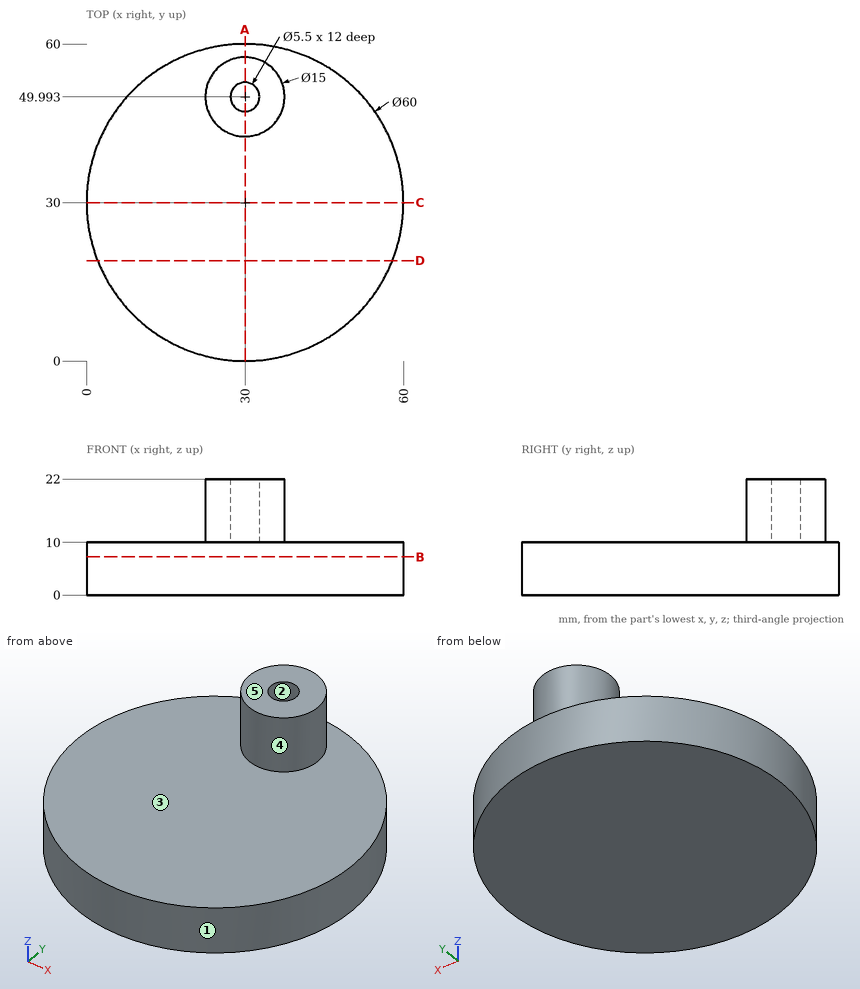
Answer from the drawing. Dimensions are ordinates in mm from the lowest x, y and z of the part. A direction names the side the tool comes from. Give positions to 0.01 mm unless a question says otherwise; leave off trailing zeros. Order: outer loops, then holes, each group sorted by start corner. A loop starts at its lowest first (then second) coordinate and runs counter-clockwise, first axis right, second up.
(1) Given pin 1 (5 mm diameter, centred on y = 32.5, z = 4, fed in from -X); pin 2 (4.5 mm diameter, centred on x = 30, y = 49.99, fed in from +Z); pin 3 (5 mm diameter, centred on y = 45.5, z = 7.5, fed in from -X); pin 4 (8 mm diameter, centred on y = 12, z = 4, fed in from -X), each flat-ended and moving along its own axis, determine where each tip first touches the part or whether it passes through.
(2) For a pull along Y with two mould halves and no side action, classify the marked faces 1, 2 and 3 as released by +Y, released by -Y, zero draft, split by the parting line, or undercut.
(3) Find section C-C (y = 30). Give the vertices of the cut face in (x, z).
(4) Find section D-D (y = 19). Give the vertices of the cut face in (x, z).
(5) Find section B-B (z = 7.25). Give the vertices of the cut face in (x, y), plus the area to 3 significant figures.
(6) Straight lines are drawn through the part: L1, parallel to Y at x = 30, z = 17; L2, parallel to Z at x = 34, y = 6.5; L3, parallel to X at y = 48, z = 18.75 (1 decimal). For each, find the intervals that lie inside material, in ascending order.
(7) Find section A-A (x = 30). Give the vertices of the cut face in (y, z).
(8) For the marked faces 4 and 5, determine the directions among +Z, -Z, +X, -X, +Y, -Y from which every point of the face is accessible in a straight line to the end or side of a thin tool.
Result sheet:
1. pin 1: stops at x = 0
1. pin 2: stops at z = 10
1. pin 3: stops at x = 2.96
1. pin 4: stops at x = 3.47
2. face 1: split by the parting line
2. face 2: undercut
2. face 3: zero draft
3. outline: (0, 0) - (60, 0) - (60, 10) - (0, 10) - close
4. outline: (2.09, 0) - (57.91, 0) - (57.91, 10) - (2.09, 10) - close
5. outline: circle Ø60 at (30, 30)
5. area: 2,830 mm2
6. L1: y = 42.49 to 47.24, 52.74 to 57.49
6. L2: z = 0 to 10
6. L3: x = 22.8 to 28.1, 31.9 to 37.2
7. outline: (0, 0) - (60, 0) - (60, 10) - (57.49, 10) - (57.49, 22) - (52.74, 22) - (52.74, 10) - (47.24, 10) - (47.24, 22) - (42.49, 22) - (42.49, 10) - (0, 10) - close
8. face 4: +Z
8. face 5: +Z, +X, -X, +Y, -Y
